Input: part model. Units: mm. Frame: model coordinates. A direction names the side the tool comes from. Coordinates: 2 decimals unless noted, no trailing zeros. Order: outer loops, then holes, each group sorted by start corner. A loop starts at its lowest first (then second) coordinate and runs counter-clockwise, first axis right, second up. Notation, with made-up numbers: (13, 80) - (67, 80) arc R31 ccw to (67, 112) - close; hole circle Ø10 at (67, -33.75). An arc over 180 degrees is marked (long way). One line per question, with ' | ' between items.
from build123d import *

# Parameters (mm, degrees)
PAD002_DEPTH       = 17.75
PAD002_DEPTH_BACK  = 17.75
POLARPATTERN_COUNT = 2
POLARPATTERN_ANGLE = 270
FILLET_R           = 0.5
PAD005_DEPTH       = 5
FILLET005_R        = 0.1
FILLET006_R        = 0.5
FILLET007_R        = 0.5
SKETCH009_W        = 2.5
SKETCH009_H        = 4
POCKET001_DEPTH    = 36.501


with BuildPart() as part:
    # Sketch003 → Pad002 (new body, two sides)
    with BuildSketch(Plane.YZ) as pad002_sk:
        Polygon((0, -17.75), (4.02, -17.75), (4.02, -11.25), (1.52, -11.25), (1.52, -13.25), (0, -13.25), align=None)
    pad002 = extrude(amount=PAD002_DEPTH) + extrude(pad002_sk.sketch, amount=-PAD002_DEPTH_BACK)

    # PolarPattern: Pad002 ×2 about axis
    polarpattern_axis = Axis((0, 0, 0), (0, 1, 0))
    for i in range(1, POLARPATTERN_COUNT):
        add(pad002.rotate(polarpattern_axis, i * POLARPATTERN_ANGLE / (POLARPATTERN_COUNT - 1)))

    # Mirrored: Pad002 across Sketch003 H_Axis
    add(pad002.mirror(Plane.XY))

    # Fillet
    fillet_edges = [part.edges().sort_by_distance(p)[0] for p in [
        (-17.75, 4.02, 14.5),
        (-17.75, 2.77, 11.25),
        (-17.75, 0.76, 13.25),
        (-17.75, 1.52, 12.25),
        (-17.75, 2.01, 17.75),
    ]]
    fillet(fillet_edges, radius=FILLET_R)

    # Sketch008 → Pad005 (join)
    with BuildSketch(Plane.ZX.offset(4.02)):
        Polygon((-18.75, 18.75), (18.75, 18.75), (18.75, -12.75), (17.75, -12.75), (17.75, 17.75), (-17.75, 17.75), (-17.75, -12.75), (-18.75, -12.75), align=None)
    extrude(amount=-PAD005_DEPTH)

    # Fillet005
    fillet005_edges = [part.edges().sort_by_distance(p)[0] for p in [
        (18.75, 4.02, 0),
        (3, 4.02, -18.75),
        (3, 4.02, 18.75),
    ]]
    fillet(fillet005_edges, radius=FILLET005_R)

    # Fillet006
    fillet006_edges = [part.edges().sort_by_distance(p)[0] for p in [
        (-17.75, 2.77, -11.25),
        (-17.75, 1.52, -12.25),
        (-17.75, 0, -15.5),
        (-17.75, 0.76, -13.25),
        (-17.75, 4.02, -14.5),
        (-17.75, 2.01, -17.75),
    ]]
    fillet(fillet006_edges, radius=FILLET006_R)

    # Fillet007
    fillet007_edges = [part.edges().sort_by_distance(p)[0] for p in [
        (-12.75, -0.98, 18.25),
        (-12.75, -0.98, -18.25),
    ]]
    fillet(fillet007_edges, radius=FILLET007_R)

    # Sketch009 → Pocket001 (cut, through all)
    with BuildSketch(Plane.YZ.offset(18.75)):
        with Locations((0.25, 0)):
            Rectangle(SKETCH009_W, SKETCH009_H)
    extrude(amount=-POCKET001_DEPTH, mode=Mode.SUBTRACT)


with BuildPart() as part_1:
    # Body001 placement: moved
    add(part.part.moved(Location((0, 0.3, 0))))


solid = part_1.part
Item 1: Section D-D on x = 16. Return the cut outline in (y, z), and give its area (3 significant figures).
Data:
outline: (-0.68, -18.75) - (4.22, -18.75) arc R0.1 ccw to (4.32, -18.65) - (4.32, 18.65) arc R0.1 ccw to (4.22, 18.75) - (-0.68, 18.75) - (-0.68, 17.75) - (0.3, 17.75) - (0.3, 2) - (1.8, 2) - (1.8, -2) - (0.3, -2) - (0.3, -17.75) - (-0.68, -17.75) - close | area: 147 mm^2
Item 2: Section B-B on y = 1.35. Return the cut outline in (x, z).
Data:
outline: (-17.75, -17.25) arc R0.5 ccw to (-17.25, -17.75) - (-12.75, -17.75) - (-12.75, -18.75) - (18.75, -18.75) - (18.75, -2) - (13.25, -2) - (13.25, -13.25) - (-17.25, -13.25) arc R0.5 ccw to (-17.75, -13.75) - close; (-17.75, 13.75) arc R0.5 ccw to (-17.25, 13.25) - (13.25, 13.25) - (13.25, 2) - (18.75, 2) - (18.75, 18.75) - (-12.75, 18.75) - (-12.75, 17.75) - (-17.25, 17.75) arc R0.5 ccw to (-17.75, 17.25) - close
Item 3: Contact query for flat-ended pins moving along their axis: P1, Ø4.5, axis at x = 1, z = 13.5, coming from the -Y side; P2, Ø1.2, axis at y = 3.5, z = 4.5, coming from the -X side; P3, Ø1.5, axis at x = 9.5, z = -1.5, coming from the +Y side; P4, Ø3, axis at x = -15, y = 3.5, coming from the -Z side. Output: stop coordinate, or through.
Data:
P1: y = 0.3 | P2: x = 11.25 | P3: through | P4: z = -17.75
Item 4: Ray query, line 1 (Z direction, x = 11.5, y = 1.45); line 2 (Z direction, x = -9, y = 1.85); line 3 (X direction, y = 3.7, z = 11). Return the intervals inside material, ascending.
Data:
line 1: -18.75 to -13.25, 13.25 to 18.75 | line 2: -18.75 to -11.25, 11.25 to 18.75 | line 3: 11.25 to 18.75
Item 5: Draft query along Z for faces 1 (the face through (-15, 2, -17.75)), 2 (the face through (2, 0, 17.75)), 3 (the face through (-15, 2, 17.75)). Return one class per face: released by +Z, released by -Z, zero draft, split by the parting line, or undercut.
Data:
face 1: released by -Z | face 2: undercut | face 3: released by +Z
Item 6: Access query for faces 4 (the face through (-3, 3, 11.25)), 5 (the face through (-12.75, 2, 18)), 6 (the face through (17, 1, -2)), 7 (the face through (17.75, 0, -10)). Directions: +Z, -Z, +X, -X, +Y, -Y. A direction counts if a zero-diameter tool reaches every point of the face in a straight line with its end or side. Return the directions, or none.
Data:
face 4: -X, +Y, -Y | face 5: +Z, -X, +Y, -Y | face 6: +X, -X, -Y | face 7: -X, -Y
Item 7: Section C-C on z = -5. Return the cut outline in (x, y), and give its area (3 significant figures).
Data:
outline: (11.25, 1.82) - (13.25, 1.82) - (13.25, 0.3) - (17.75, 0.3) - (17.75, -0.68) - (18.75, -0.68) - (18.75, 4.22) arc R0.1 ccw to (18.65, 4.32) - (11.25, 4.32) - close | area: 28.1 mm^2
Item 8: Section A-A on x = -4. Return the cut outline in (y, z), and give its area (3 significant figures).
Data:
outline: (-0.68, -18.75) - (4.22, -18.75) arc R0.1 ccw to (4.32, -18.65) - (4.32, -11.25) - (1.82, -11.25) - (1.82, -13.25) - (0.3, -13.25) - (0.3, -17.75) - (-0.68, -17.75) - close; (-0.68, 17.75) - (0.3, 17.75) - (0.3, 13.25) - (1.82, 13.25) - (1.82, 11.25) - (4.32, 11.25) - (4.32, 18.65) arc R0.1 ccw to (4.22, 18.75) - (-0.68, 18.75) - close | area: 56.2 mm^2
